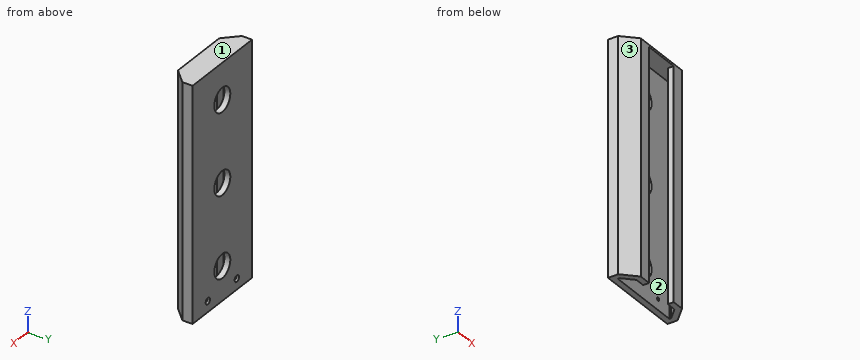
```python
from build123d import *

# Parameters (mm, degrees)
BOSS_EXTRUDE2_DEPTH = 213
BOSS_EXTRUDE4_DEPTH = 2
SKETCH4_R           = 1.5
CUT_EXTRUDE1_DEPTH  = 10
CHAMFER2_SIZE       = 1.5
SKETCH5_R           = 11
CUT_EXTRUDE2_DEPTH  = 52


with BuildPart() as part:
    # Sketch1 → Boss-Extrude2 (new body)
    with BuildSketch(Plane.XY):
        Polygon((23.240231027, 8.911538462), (23.240231027, 14.411538462), (14.033124245, 14.411538462), (4.740231027, 23.70443168), (4.740231027, 25.411538462), (75.740231027, 25.411538462), (75.740231027, 23.70443168), (66.447337808, 14.411538462), (57.240231027, 14.411538462), (57.240231027, 8.911538462), (68.725512401, 8.911538462), (81.240231027, 21.426257087), (81.240231027, 30.911538462), (-0.759768973, 30.911538462), (-0.759768973, 21.426257087), (11.754949652, 8.911538462), align=None)
    extrude(amount=BOSS_EXTRUDE2_DEPTH)

    # Sketch3 → Boss-Extrude4 (add)
    with BuildSketch(Plane.XY.offset(213)):
        Polygon((-0.759768973, 30.911538462), (-0.759768973, 21.426257087), (11.754949652, 8.911538462), (23.240231027, 8.911538462), (57.240231027, 8.911538462), (68.725512401, 8.911538462), (81.240231027, 21.426257087), (81.240231027, 30.911538462), align=None)
    extrude(amount=BOSS_EXTRUDE4_DEPTH)

    # Sketch4 → Cut-Extrude1 (cut)
    with BuildSketch(Plane(origin=(0, 30.911538462, 0), x_dir=(1, 0, 0), z_dir=(0, 1, 0))):
        with Locations(Location((60.240231027, -10, 0), (0, 0, 180))):
            Circle(SKETCH4_R)
        with Locations(Location((20.240231027, -10, 0), (0, 0, 270))):
            Circle(SKETCH4_R)
    extrude(amount=-CUT_EXTRUDE1_DEPTH, mode=Mode.SUBTRACT)

    # Chamfer2
    chamfer2_edges = [part.edges().sort_by_distance(p)[0] for p in [
        (61.740231027, 30.911538462, 10),
        (20.240231027, 30.911538462, 8.5),
    ]]
    chamfer(chamfer2_edges, length=CHAMFER2_SIZE)

    # Sketch5 → Cut-Extrude2 (cut)
    with BuildSketch(Plane(origin=(0, 30.911538462, 0), x_dir=(1, 0, 0), z_dir=(0, 1, 0))):
        with Locations(Location((40.240231027, -31.5, 0), (0, 0, 180))):
            Circle(SKETCH5_R)
        with Locations(Location((40.240231027, -106.5, 0), (0, 0, 180))):
            Circle(SKETCH5_R)
        with Locations(Location((40.240231027, -181.5, 0), (0, 0, 180))):
            Circle(SKETCH5_R)
    extrude(amount=-CUT_EXTRUDE2_DEPTH, mode=Mode.SUBTRACT)


solid = part.part
```
Work out the finished part from the listing and answer in its coordinate system (mm). Face numbers are marked on the shaded views. Coordinates: 2 decimals unless noted, no trailing zeros. Write each loop counter-clockwise with the first axis right and the second up, starting at its lowest first coordinate (ties: lowest second). Pieces come first, ordered by that corner, then holes. Notation, with made-up numbers: (-22, 16.5) - (-5, 16.5) arc R14 cw to (-5, 20.5) - close; hole circle Ø5 at (-19.75, 30.5). An arc over 180 degrees is marked (long way). Answer as a JSON object with one key per item and string values.
Q1. Given pin 1 Ø1.6 at (y, z) = (12.5, 101.5) entering from -X; pin 2 Ø1.8 at (x, z) = (60.24, 10) entering from +Y; pin 3 Ø10 at (y, z) = (11.5, 131.5) entering from +X, each flat-ended and moving along its own axis, determine where each tip first touches the part or whether it passes through.
Results list:
{"pin 1": "stops at x = 7.37", "pin 2": "stops at y = 14.41", "pin 3": "stops at x = 76.31"}
Q2. Find section A-A (z = 31.5). Write down the section's boundary in (x, y), plus the area to 3 significant figures.
Results list:
{"outline": "(-0.76, 21.43) - (11.75, 8.91) - (23.24, 8.91) - (23.24, 14.41) - (14.03, 14.41) - (4.74, 23.7) - (4.74, 25.41) - (29.24, 25.41) - (29.24, 30.91) - (-0.76, 30.91) - close; (51.24, 25.41) - (75.74, 25.41) - (75.74, 23.7) - (66.45, 14.41) - (57.24, 14.41) - (57.24, 8.91) - (68.73, 8.91) - (81.24, 21.43) - (81.24, 30.91) - (51.24, 30.91) - close", "area": "645 mm^2"}
Q3. For a pull along Y with two mould halves and no side action, classify the marked faces 1, 2 and 3 as pulls with the +Y half, pulls with the -Y half, needs draft (parallel to the pull), parting line crosses it, or undercut.
Results list:
{"face 1": "needs draft", "face 2": "undercut", "face 3": "pulls with the -Y half"}
Q4. Consider L1, parallel to X at y = 25.25, z = 9; L2, parallel to Y at x = 14, z = 130.5; L3, parallel to Z at x = 44.5, y = 29.75. Determine where each line is inside the solid, lowest interval first. Write a range as from..to.
Results list:
{"L1": "x = -0.76..4.74, 75.74..81.24", "L2": "y = 8.91..14.44, 25.41..30.91", "L3": "z = 0..21.36, 41.64..96.36, 116.64..171.36, 191.64..215"}
Q5. Find section D-D (x = 55). Write down the section's boundary in (y, z).
Results list:
{"outline": "(8.91, 213) - (25.41, 213) - (25.41, 0) - (30.91, 0) - (30.91, 215) - (8.91, 215) - close"}
Q6. Find section B-B (x = 43). Write down the section's boundary in (y, z), plus the area to 3 significant figures.
Results list:
{"outline": "(8.91, 213) - (25.41, 213) - (25.41, 192.15) - (30.91, 192.15) - (30.91, 215) - (8.91, 215) - close; (25.41, 0) - (30.91, 0) - (30.91, 20.85) - (25.41, 20.85) - close; (25.41, 42.15) - (30.91, 42.15) - (30.91, 95.85) - (25.41, 95.85) - close; (25.41, 117.15) - (30.91, 117.15) - (30.91, 170.85) - (25.41, 170.85) - close", "area": "864 mm^2"}
Q7. Find section C-C (z = 91). Write down the section's boundary in (x, y), plus the area to 3 significant figures.
Results list:
{"outline": "(-0.76, 21.43) - (11.75, 8.91) - (23.24, 8.91) - (23.24, 14.41) - (14.03, 14.41) - (4.74, 23.7) - (4.74, 25.41) - (75.74, 25.41) - (75.74, 23.7) - (66.45, 14.41) - (57.24, 14.41) - (57.24, 8.91) - (68.73, 8.91) - (81.24, 21.43) - (81.24, 30.91) - (-0.76, 30.91) - close", "area": "766 mm^2"}
